Check sheet for the drawn part. Datum: minimum x, y, z corner. Units: mm. Round coordinates to 2 decimals unless told otherwise and drop trailing zeros. Order: outer loops, then holes, each group sorted by start corner. A loop starts at its lowest first (then second) coordinate and runs counter-clockwise, first axis right, second up. Notation, with made-up numbers: M -12.75,80 L 19.25,80 A21 ccw 19.25,119 Z; hole C 22,38 d5. An arc over 180 degrees is marked long. Use one line per item in the form item = value. Start each with the question number.
Item 1: Cross-section at D-D on y = 26. Enter the section's corners in (x, z).
Item 2: Go/stop test with flat-tipped pins: pin 1 Ø8 at (x, z) = (12, 22) entering from -Y; pin 2 Ø1.5 at (y, z) = (17.5, 88) entering from +X; pin 3 Ø1 at (x, z) = (12.5, 22.5) entering from +Y; pin 4 Ø5 at (x, z) = (22, 19.5) entering from -Y. Record where each tip stops, or that it passes through.
Item 3: Thickness scan on probe 1 along X at (y, z) = (14.25, 11); probe 2 along Y at (x, z) = (14, 68); probe 3 along X at (y, z) = (17.5, 57). Record the ranges inside material, lowest first. Write a range as [from, to].
Item 4: Cross-section at A-A on y = 14. Enter the section's corners in (x, z).
Item 5: Cross-section at C-C on z = 93. Enter the section's corners in (x, y).
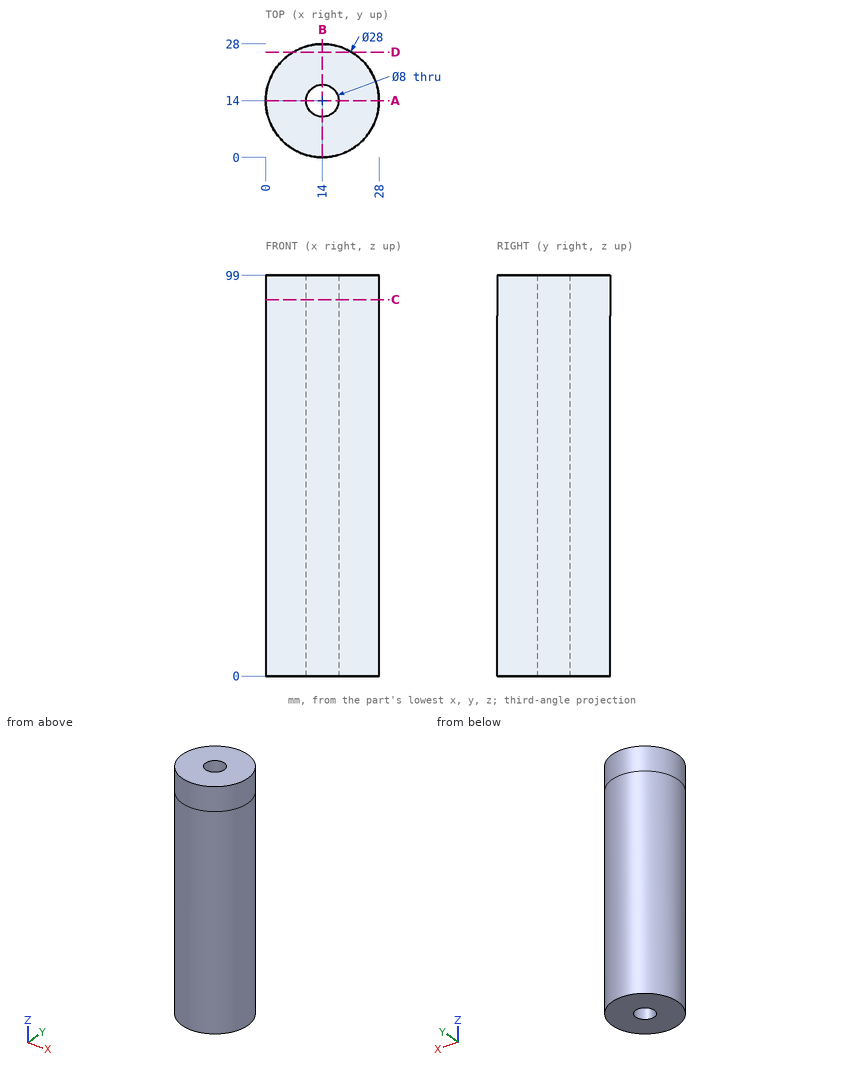
Output values:
q1.outline = M 6.79,0 L 21.21,0 L 21.21,99 L 6.79,99 Z
q2.pin_1 = 0
q2.pin_2 = 27.73
q2.pin_3 = 27.96
q2.pin_4 = 1.13
q3.probe_1 = [0, 10.01], [17.99, 28]
q3.probe_2 = [0, 10], [18, 28]
q3.probe_3 = [0.44, 12.06], [15.94, 27.56]
q4.outline = M 0,0 L 10,0 L 10,99 L 0,99 Z; M 18,0 L 28,0 L 28,99 L 18,99 Z
q5.outline = C 14,14 d28; hole C 14,14 d8
